Read the model definition and answer for the solid it produces. Units are mm, in the model's axes. A direction names the side the tool comes from. Coordinates: 2 decimals unless noted, no trailing zeros. Order: outer loops, then holes, each group sorted by start corner. A loop starts at its lowest first (then second) coordinate and runs counter-clockwise, first axis right, second up. Notation, with made-up numbers: (57, 43.25) - (105, 43.25) arc R24 cw to (105, 74.25) - close; hole circle Ø9 at (36.5, 27.5). An arc over 180 degrees is marked (long way). Write item = value, one per line.
from build123d import *

# Parameters (mm, degrees)
SKETCH1_R           = 1.575
BOSS_EXTRUDE1_DEPTH = 9.525
CUT_EXTRUDE4_REACH  = 11.525
SKETCH2_W           = 3.205
SKETCH2_H           = 10
SKETCH4_R           = 1.190625
CUT_EXTRUDE5_DEPTH  = 1.75


with BuildPart() as part:
    # Sketch1 → Boss-Extrude1 (new body)
    with BuildSketch(Plane.XY):
        with BuildLine():
            Line((4.7625, 9.25), (4.7625, 1.75))
            Line((4.7625, 1.75), (12.7625, 1.75))
            Line((12.7625, 1.75), (12.7625, 0))
            Line((12.7625, 0), (0, 0))
            ThreePointArc((0, 0), (-3.501964629, 4.047983414), (-4.7625, 9.25))
            ThreePointArc((-4.7625, 9.25), (0, 14.0125), (4.7625, 9.25))
        make_face()
        with Locations((0, 9.25)):
            Circle(SKETCH1_R, mode=Mode.SUBTRACT)
    extrude(amount=BOSS_EXTRUDE1_DEPTH)

    # Sketch2 → Cut-Extrude4 (cut, up to next)
    with BuildSketch(Plane.ZY.offset(-4.7625), mode=Mode.PRIVATE) as cut_extrude4_sk1:
        with Locations((4.7625, 9.0125)):
            Rectangle(SKETCH2_W, SKETCH2_H)
    cut_extrude4_tool1 = extrude(cut_extrude4_sk1.sketch, amount=CUT_EXTRUDE4_REACH, mode=Mode.PRIVATE) & part.part
    add(cut_extrude4_tool1.solids().sort_by_distance((4.7625, 9.0125, 4.7625))[0], mode=Mode.SUBTRACT)

    # Sketch4 → Cut-Extrude5 (cut)
    with BuildSketch(Plane(origin=(0, 1.75, 0), x_dir=(1, 0, 0), z_dir=(0, 1, 0))):
        with BuildLine():
            Line((12.7625, -9.525), (12.7625, -4.7625))
            ThreePointArc((12.7625, -4.7625), (11.62983327, -7.872218888), (8.7625, -9.525))
            Line((8.7625, -9.525), (12.7625, -9.525))
        make_face()
        with BuildLine():
            Line((12.7625, 0), (8.7625, 0))
            ThreePointArc((8.7625, 0), (11.62983327, -1.652781112), (12.7625, -4.7625))
            Line((12.7625, -4.7625), (12.7625, 0))
        make_face()
        with Locations((8.7625, -4.7625)):
            Circle(SKETCH4_R)
    extrude(amount=-CUT_EXTRUDE5_DEPTH, mode=Mode.SUBTRACT)


solid = part.part
1) For faces 1 (the face through (1.1, 7.8, 3.16)), 2 (the face through (-0.1, 14.01, 1.56)), 3 (the face through (4.762, 3, 5)), determine the directions among +Z, -Z, +X, -X, +Y, -Y from which every point of the face is accessible in a straight line to the end or side of a thin tool.
Returned:
face_1 = +X, -X, +Y
face_2 = +Z, -Z, +Y
face_3 = +Z, -Z, +X, +Y
2) Determine the mould class of faces 4 (the face through (1, 7, 9.525)), 5 (the face through (9.898, 0.887, 4.405)), 6 (the face through (1.1, 7.8, 6.365)), 7 (the face through (8, 1.75, 6)) for opening direction Z: pulls with the +Z half, pulls with the -Z half, needs draft (parallel to the pull), parting line crosses it, or undercut.
Returned:
face_4 = pulls with the +Z half
face_5 = undercut
face_6 = undercut
face_7 = needs draft
3) The part is cut by section B-B (y = 12.5). Determine the outline of the cut face in (x, z) (3 decimals).
Returned:
outline = (-3.481, 0) - (3.481, 0) - (3.481, 3.16) - (-3.481, 3.16) - close; (-3.481, 6.365) - (3.481, 6.365) - (3.481, 9.525) - (-3.481, 9.525) - close
4) Straight lines are drawn through the part: line 1 along X through (y, z) = (9.25, 0.7) (1 decimal); line 2 along Z through (x, y) = (3.25, 6.5) (3 decimals); line 3 along Y through (x, z) = (10, 8.75). For each, find the intervals that lie inside material, in ascending order. Write a range as from..to.
Returned:
line_1 = -4.8..-1.6, 1.6..4.8
line_2 = 0..3.16, 6.365..9.525
line_3 = 0..1.75
5) The part is cut by section A-A (z = 4). Determine the outline of the cut face in (x, y).
Returned:
outline = (-3.48, 4.01) arc R11.36 ccw to (0, 0) - (7.85, 0) - (7.85, 1.75) - (4.76, 1.75) - (4.76, 4.01) - close; (9.68, 0) - (12.7, 0) - (12.7, 1.75) - (9.68, 1.75) - close
6) Flat-ended cylindrical pins translate along their axes: pin 1 Ø2.5 at (x, y) = (0, 9.25) entering from -Z (1 decimal); pin 2 Ø4 at (y, z) = (7, 7) entering from +X; pin 3 Ø1.5 at (x, z) = (8, 2.5) entering from +Y; pin 4 Ø1 at (x, z) = (0.5, 5.5) entering from +Y. Find the tip coordinate at first contact, or state that the pin passes through.
Returned:
pin_1 = through
pin_2 = 4.76
pin_3 = 1.75
pin_4 = 4.01
7) The part is cut by section C-C (x = -1.25). Determine the outline of the cut face in (y, z) (1 decimal).
Returned:
outline = (1, 0) - (8.3, 0) - (8.3, 3.2) - (4, 3.2) - (4, 6.4) - (8.3, 6.4) - (8.3, 9.5) - (1, 9.5) - close; (10.2, 0) - (13.8, 0) - (13.8, 3.2) - (10.2, 3.2) - close; (10.2, 6.4) - (13.8, 6.4) - (13.8, 9.5) - (10.2, 9.5) - close
